For this review, use the dimensioned drawing (mm, ordinates from the lowest corner) and the shaded views. A direction names the side the tool comes from. Round coordinates to 2 decimals unless told otherwise and drop trailing zeros. Write each loop counter-clockwise with the first axis right and the second up, starting at its lowest first coordinate (ties: lowest second). Pieces come first, ordered by that corner, then holes. Notation, with made-up numbers: (29, -13.5) - (37, -13.5) arc R31 cw to (37, 23.5) - close; hole circle Ø9 at (81, -15). An arc over 180 degrees is marked (long way). Return JSON: item names as keys, results as strings.
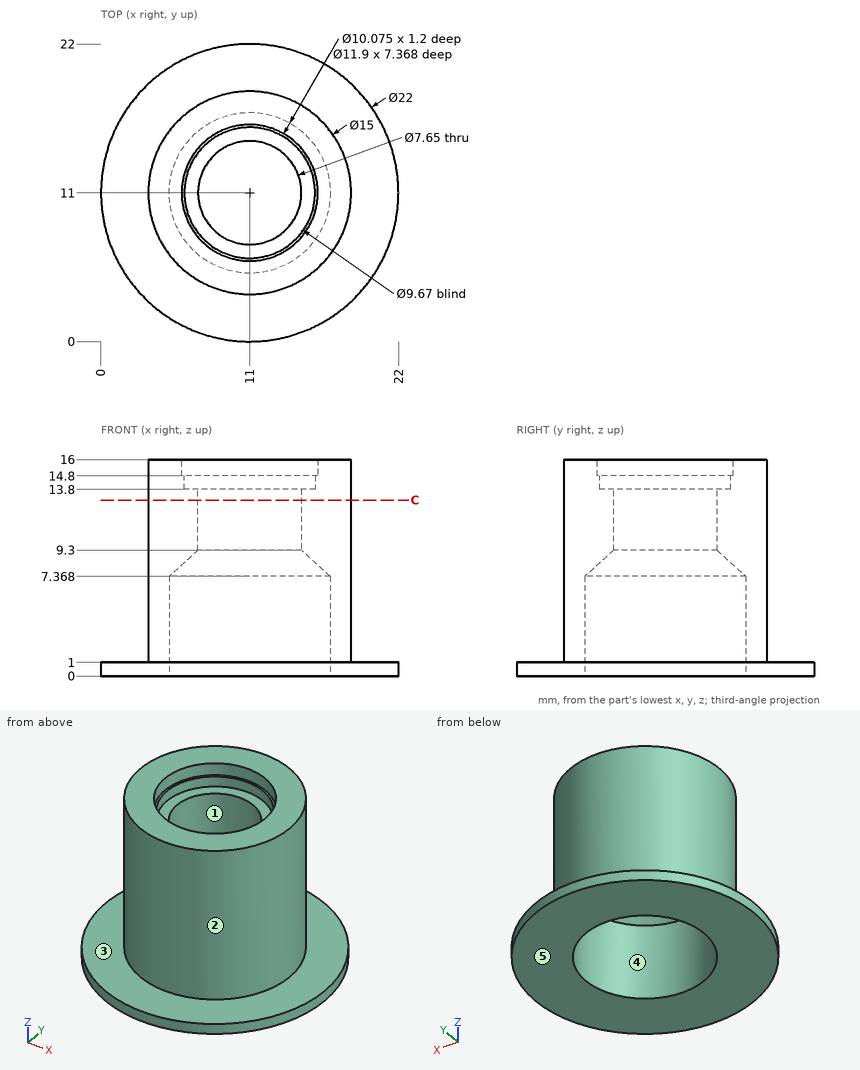
(1) Mouldability with a two-part tool opening along X and no side actions: class the marked faces 1, 2 and 3 as released by +X, released by -X, zero draft, split by the parting line, or undercut.
Filled in:
{"face 1": "undercut", "face 2": "split by the parting line", "face 3": "zero draft"}
(2) Add section C-C (z = 13). Write out the cut boundary in (x, y) (3 decimals).
Filled in:
{"outline": "circle Ø15 at (11, 11); hole circle Ø7.65 at (11, 11)"}
(3) For the marked faces 4 and 5, list the 3-axis set-ups (+Z, -Z, +X, -X, +Y, -Y) from which the entire face can be reached by the end or side of a thin tool; tool diameter is ignored.
Filled in:
{"face 4": "-Z", "face 5": "-Z, +X, -X, +Y, -Y"}
(4) Clearance check with flat-ended pins moving along their axes: pin 1 Ø4 at (y, z) = (19.5, 11.5) entering from -X; pin 2 Ø5 at (x, y) = (10.5, 13.5) entering from -Z; pin 3 Ø2 at (x, z) = (3.5, 3.5) entering from +Y; pin 4 Ø6 at (x, y) = (11, 11) entering from -Z. State where each tip first meets the part, or that it passes through.
Filled in:
{"pin 1": "stops at x = 7.26", "pin 2": "stops at z = 8.19", "pin 3": "stops at y = 14.74", "pin 4": "passes through"}
(5) Wall thickness on line 1 (Y direction, x = 11, z = 10.7) (3 decimals); line 2 (Y direction, x = 11, z = 5.5); line 3 (Z direction, x = 20, y = 8.5): over which ranges is each line inside the solid? List them lowest first.
Filled in:
{"line 1": "y = 3.5 to 7.175, 14.825 to 18.5", "line 2": "y = 3.5 to 5.05, 16.95 to 18.5", "line 3": "z = 0 to 1"}
